Work out the finished part from the listing and answer in its coordinate system (mm). Give positions to 0.01 mm unless a question says otherwise; leave off trailing zeros. Order: outer loops, then holes, each group sorted by start corner. A loop starts at its lowest first (then second) coordinate and runs counter-clockwise, first axis right, second up. Notation, with made-up numbers: (86.25, 82) -> (102.25, 82) arc R14 ccw to (102.25, 102) -> close; hole circle Ø4 at (63.5, -38). An arc over 180 degrees is marked (long way). Answer as CSV lines item,"result". Start each with the question number.
1. Find the intervals of material crossed by L1, parallel to Z at x = 92.5, y = -16.5, in increasing order.
2. A cutting plane is placed at A-A (y = -13.25). Give the vertices of the cut face in (x, z).
3. Flat-ended cylindrical pins translate along their axes: pin 1 (21 mm diameter, centred on x = 88.5, z = 566, fed in from -Y); pin 2 (5 mm diameter, centred on x = 238, y = -12.5, fed in from -Z); pin 3 (7.5 mm diameter, centred on x = 113, y = -13.5, fed in from +Z); pin 4 (5.5 mm diameter, centred on x = 167.5, z = 187, fed in from -Y) (3 decimals). Find the tip coordinate at first contact, or state that the pin passes through.
4. A cutting plane is placed at B-B (x = 189). Give the vertices of the cut face in (y, z) (3 decimals).
from build123d import *

# Parameters (mm, degrees)
F0_W      = 317.5
F0_H      = 1346.2
F1_DEPTH  = 19.05
F2_W      = 317.5
F2_H      = 9.525
F3_DEPTH  = 19.05
F4_W      = 317.5
F4_H      = 9.525
F5_DEPTH  = 19.05
F6_W      = 317.5
F6_H      = 19.05
F7_DEPTH  = 9.525
F8_W      = 317.5
F8_H      = 19.05
F9_DEPTH  = 9.525
F10_W     = 317.5
F10_H     = 19.05
F11_DEPTH = 9.525


with BuildPart() as f1:
    # F0 (on Front) → F1 (new body)
    with BuildSketch(Plane.XZ):
        with Locations((158.75, 673.1)):
            Rectangle(F0_W, F0_H)
    extrude(amount=F1_DEPTH)

    # F2 (on face) → F3 (cut)
    with BuildSketch(Plane.XY.offset(1346.2)):
        with Locations((158.75, -14.2875)):
            Rectangle(F2_W, F2_H)
    extrude(amount=-F3_DEPTH, mode=Mode.SUBTRACT)

    # F4 (on face) → F5 (cut)
    with BuildSketch(Plane(origin=(0, 0, 0), x_dir=(1, 0, 0), z_dir=(0, 0, -1))):
        with Locations((158.75, 14.2875)):
            Rectangle(F4_W, F4_H)
    extrude(amount=-F5_DEPTH, mode=Mode.SUBTRACT)

    # F6 (on face) → F7 (cut)
    with BuildSketch(Plane.XZ.offset(19.05)):
        with Locations((158.75, 187.325)):
            Rectangle(F6_W, F6_H)
    extrude(amount=-F7_DEPTH, mode=Mode.SUBTRACT)

    # F8 (on face) → F9 (cut)
    with BuildSketch(Plane.XZ.offset(19.05)):
        with Locations((158.75, 568.325)):
            Rectangle(F8_W, F8_H)
    extrude(amount=-F9_DEPTH, mode=Mode.SUBTRACT)

    # F10 (on face) → F11 (cut)
    with BuildSketch(Plane.XZ.offset(19.05)):
        with Locations((158.75, 949.325)):
            Rectangle(F10_W, F10_H)
    extrude(amount=-F11_DEPTH, mode=Mode.SUBTRACT)


solid = f1.part
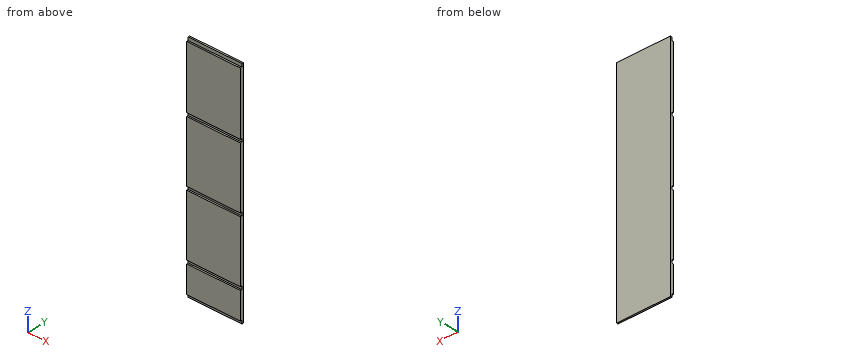
Answer sheet:
1,L1,"z = 19.05 to 177.8, 196.85 to 558.8, 577.85 to 939.8, 958.85 to 1327.15"
2,outline,"(0, 19.05) -> (317.5, 19.05) -> (317.5, 177.8) -> (0, 177.8) -> close; (0, 196.85) -> (317.5, 196.85) -> (317.5, 558.8) -> (0, 558.8) -> close; (0, 577.85) -> (317.5, 577.85) -> (317.5, 939.8) -> (0, 939.8) -> close; (0, 958.85) -> (317.5, 958.85) -> (317.5, 1327.15) -> (0, 1327.15) -> close"
3,pin 1,"stops at y = -19.05"
3,pin 2,"stops at z = 19.05"
3,pin 3,"stops at z = 1327.15"
3,pin 4,"stops at y = -9.525"
4,outline,"(-19.05, 19.05) -> (-9.525, 19.05) -> (-9.525, 0) -> (0, 0) -> (0, 1346.2) -> (-9.525, 1346.2) -> (-9.525, 1327.15) -> (-19.05, 1327.15) -> (-19.05, 958.85) -> (-9.525, 958.85) -> (-9.525, 939.8) -> (-19.05, 939.8) -> (-19.05, 577.85) -> (-9.525, 577.85) -> (-9.525, 558.8) -> (-19.05, 558.8) -> (-19.05, 196.85) -> (-9.525, 196.85) -> (-9.525, 177.8) -> (-19.05, 177.8) -> close"
